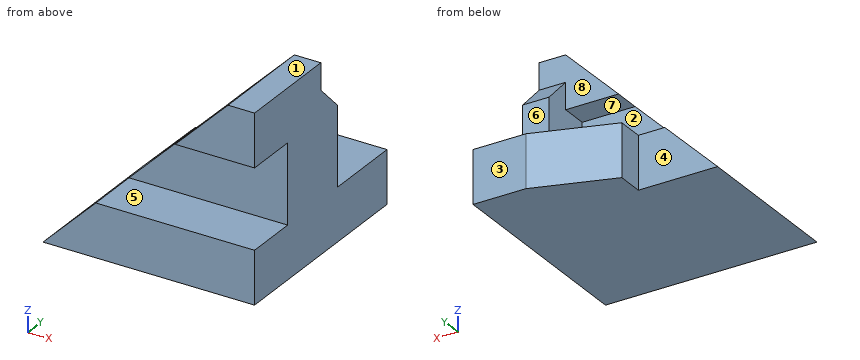
from build123d import *

# Parameters (mm, degrees)
SKETCH1_W           = 40
SKETCH1_H           = 40
BOSS_EXTRUDE1_DEPTH = 10
CUT_EXTRUDE1_DEPTH  = 11
CUT_EXTRUDE2_DEPTH  = 11
SKETCH4_W           = 40
SKETCH4_H           = 20
BOSS_EXTRUDE2_DEPTH = 25
SKETCH5_W           = 15
SKETCH5_H           = 5
CUT_EXTRUDE3_DEPTH  = 41
SKETCH7_W           = 15
SKETCH7_H           = 10
CUT_EXTRUDE4_DEPTH  = 41
CUT_EXTRUDE5_DEPTH  = 31
SKETCH9_W           = 5
SKETCH9_H           = 10
BOSS_EXTRUDE3_DEPTH = 20
CUT_EXTRUDE6_DEPTH  = 6


with BuildPart() as part:
    # Sketch1 → Boss-Extrude1 (new body)
    with BuildSketch(Plane.XY):
        Rectangle(SKETCH1_W, SKETCH1_H)
    extrude(amount=BOSS_EXTRUDE1_DEPTH)

    # Sketch2 → Cut-Extrude1 (cut, through all)
    with BuildSketch(Plane.XY.offset(10)):
        Polygon((10, 20), (-5, 15), (-5, 20), align=None)
    extrude(amount=-CUT_EXTRUDE1_DEPTH, mode=Mode.SUBTRACT)

    # Sketch3 → Cut-Extrude2 (cut, through all)
    with BuildSketch(Plane.XY.offset(10)):
        Polygon((-5, 15), (-5, 10), (-20, 10), (-20, 20), (-5, 20), align=None)
    extrude(amount=-CUT_EXTRUDE2_DEPTH, mode=Mode.SUBTRACT)

    # Sketch4 → Boss-Extrude2 (add)
    with BuildSketch(Plane.XY.offset(10)):
        with Locations((0, -10)):
            Rectangle(SKETCH4_W, SKETCH4_H)
    extrude(amount=BOSS_EXTRUDE2_DEPTH)

    # Sketch5 → Cut-Extrude3 (cut, through all)
    with BuildSketch(Plane.ZY.offset(20)):
        with Locations((17.5, -2.5)):
            Rectangle(SKETCH5_W, SKETCH5_H)
    extrude(amount=-CUT_EXTRUDE3_DEPTH, mode=Mode.SUBTRACT)

    # Sketch7 → Cut-Extrude4 (cut, through all)
    with BuildSketch(Plane.ZY.offset(20)):
        with Locations((17.5, -15)):
            Rectangle(SKETCH7_W, SKETCH7_H)
    extrude(amount=-CUT_EXTRUDE4_DEPTH, mode=Mode.SUBTRACT)

    # Sketch8 → Cut-Extrude5 (cut, through all)
    with BuildSketch(Plane(origin=(0, 10, 0), x_dir=(1, 0, 0), z_dir=(0, 1, 0))):
        Polygon((-20, 0), (15, -35), (-20, -35), align=None)
    extrude(amount=-CUT_EXTRUDE5_DEPTH, mode=Mode.SUBTRACT)

    # Sketch9 → Boss-Extrude3 (add)
    with BuildSketch(Plane.XY.offset(10)):
        with Locations((17.5, 0)):
            Rectangle(SKETCH9_W, SKETCH9_H)
    extrude(amount=BOSS_EXTRUDE3_DEPTH)

    # Sketch10 → Cut-Extrude6 (cut, through all)
    with BuildSketch(Plane.ZY.offset(-15)):
        Polygon((30, 0), (25, 5), (30, 5), align=None)
    extrude(amount=-CUT_EXTRUDE6_DEPTH, mode=Mode.SUBTRACT)


solid = part.part
The listing builds one solid part. Answer for the finished solid, in the listing's coordinates (mm). Face numbers are marked on the shaded views. A direction names the side the tool comes from. Coordinates: 2 decimals unless noted, no trailing zeros. Order: outer loops, then holes, each group sorted by start corner. A loop starts at its lowest first (then second) coordinate and runs counter-clockwise, first axis right, second up.
Q1. A cutting plane is placed at A-A, the plane y = -11. Write down the section's boundary in (x, z), and give its area (3 significant figures).
Q2. Consider line 1 (Z direction, x = 1.5, y = -3.5); line 2 (Y direction, x = 14.5, z = 31); line 3 (Y direction, x = 9, z = 17.5). Determine where each line is inside the solid, lowest interval first.
Q3. A cutting plane is placed at C-C, the plane z = 19. Write down the section's boundary in (x, y).
Q4. A cutting plane is placed at B-B, the plane x = 7. Write down the section's boundary in (y, z).
Q5. Which of the six approach directions +Z, -Z, +X, -X, +Y, -Y give full straight-line access (tool end or side, diameter ignored) to the marked faces 4, 5, 6, 7 and 8?
Q6. Given P1, Ø11, axis at x = 14.5, z = 28, coming from the +Y side; P2, Ø5, axis at y = -3.5, z = 22, coming from the -X side; P3, Ø5, axis at x = -14.5, z = 6.5, coming from the +Y side; P4, Ø5, axis at x = 15, y = -17, coming from the -Z side, each flat-ended and moving along its own axis, determine where each tip first touches the part or whether it passes through.
Q7. For a pull along Z with two mould halves and no side action, classify the marked faces 1, 2 and 3 as pulls with the +Z half, pulls with the -Z half, needs draft (parallel to the pull), parting line crosses it, or undercut.
Q8. A cutting plane is placed at D-D, the plane y = -3.5. Write down the section's boundary in (x, z), and give its area (3 significant figures).
Answers follow:
1. outline: (-20, 0) - (20, 0) - (20, 10) - (-10, 10) - close; (5, 25) - (20, 25) - (20, 35) - (15, 35) - close
1. area: 450 mm2
2. line 1: z = 0 to 10
2. line 2: y = -20 to 0
2. line 3: y = -10 to -5
3. outline: (-1, -10) - (20, -10) - (20, 5) - (15, 5) - (15, -5) - (-1, -5) - close
4. outline: (-20, 0) - (19, 0) - (19, 10) - (-5, 10) - (-5, 25) - (0, 25) - (0, 27) - (-20, 27) - (-20, 25) - (-10, 25) - (-10, 10) - (-20, 10) - close
5. face 4: +Z, -Z, -X, +Y
5. face 5: +X, -X, -Y
5. face 6: +Z, +X, -X, +Y
5. face 7: -X, +Y
5. face 8: +Z, -X, +Y
6. P1: stops at y = 5
6. P2: stops at x = 0
6. P3: stops at y = 10
6. P4: stops at z = 0
7. face 1: pulls with the +Z half
7. face 2: undercut
7. face 3: needs draft
8. outline: (-20, 0) - (20, 0) - (20, 35) - (15, 35) - (5, 25) - (15, 25) - (15, 10) - (-10, 10) - close
8. area: 525 mm2
